Verification items for the finished model (mm, model axes). A direction names the side the tool comes from. Round coordinates to 2 decimals unless told otherwise and drop trailing zeros. Order: outer loops, then holes, each group sorted by start corner. A loop starts at its lowest first (then second) coordinate and runs counter-clockwise, first axis right, second up.
```python
from build123d import *

# Parameters (mm, degrees)
CROQUIS1_W              = 50
CROQUIS1_H              = 97
SALIENTE_EXTRUIR1_DEPTH = 5
CORTAR_EXTRUIR1_DEPTH   = 6
CROQUIS2_R              = 3.6
CROQUIS2_R_2            = 2.55
CORTAR_EXTRUIR2_DEPTH   = 6
CROQUIS4_R              = 6
CROQUIS4_R_2            = 5.05
CORTAR_EXTRUIR3_DEPTH   = 2
REDONDEO1_R             = 5
CROQUIS5_R              = 1.55
CROQUIS5_W              = 6
CROQUIS5_H              = 4.2
CORTAR_EXTRUIR4_DEPTH   = 6
CORTAR_EXTRUIR6_DEPTH   = 6
CROQUIS14_R             = 3
CORTAR_EXTRUIR9_DEPTH   = 2.5
CROQUIS18_R             = 10.5
CROQUIS18_R_2           = 1.525
CORTAR_EXTRUIR10_DEPTH  = 6


with BuildPart() as part:
    # Croquis1 → Saliente-Extruir1 (new body)
    with BuildSketch(Plane(origin=(0, 0, 0), x_dir=(1, 0, 0), z_dir=(0, 1, 0))):
        Rectangle(CROQUIS1_W, CROQUIS1_H)
    extrude(amount=SALIENTE_EXTRUIR1_DEPTH)

    # Croquis3 → Cortar-Extruir1 (cut, through all)
    with BuildSketch(Plane(origin=(0, 5, 0), x_dir=(1, 0, 0), z_dir=(0, 1, 0))):
        with BuildLine():
            Line((-14.1, -41.5), (-14.1, -48.5))
            Line((-14.1, -48.5), (-25, -48.5))
            Line((-25, -48.5), (-25, -28.05))
            ThreePointArc((-25, -28.05), (-17.369189497, -33.007651712), (-14.1, -41.5))
        make_face()
        with BuildLine():
            Line((25, -48.5), (14.1, -48.5))
            Line((14.1, -48.5), (14.1, -41.5))
            ThreePointArc((14.1, -41.5), (17.369189497, -33.007651712), (25, -28.05))
            Line((25, -28.05), (25, -48.5))
        make_face()
    extrude(amount=-CORTAR_EXTRUIR1_DEPTH, mode=Mode.SUBTRACT)

    # Croquis2 → Cortar-Extruir2 (cut, through all)
    with BuildSketch(Plane(origin=(0, 5, 0), x_dir=(1, 0, 0), z_dir=(0, 1, 0))):
        with Locations((-15, 32.45)):
            Circle(CROQUIS2_R)
        with Locations((15, 32.45)):
            Circle(CROQUIS2_R)
        with Locations((15, -19.45)):
            Circle(CROQUIS2_R_2)
        with Locations((-15, -19.45)):
            Circle(CROQUIS2_R_2)
    extrude(amount=-CORTAR_EXTRUIR2_DEPTH, mode=Mode.SUBTRACT)

    # Croquis4 → Cortar-Extruir3 (cut)
    with BuildSketch(Plane.XZ):
        with Locations((15, -32.45)):
            Circle(CROQUIS4_R)
        with Locations((-15, -32.45)):
            Circle(CROQUIS4_R)
        with Locations((-15, 19.45)):
            Circle(CROQUIS4_R_2)
        with Locations((15, 19.45)):
            Circle(CROQUIS4_R_2)
    extrude(amount=-CORTAR_EXTRUIR3_DEPTH, mode=Mode.SUBTRACT)

    # Redondeo1
    redondeo1_edges = [part.edges().sort_by_distance(p)[0] for p in [
        (-25, 2.5, 28.05),
        (25, 2.5, 28.05),
        (-25, 2.5, -48.5),
        (25, 2.5, -48.5),
    ]]
    fillet(redondeo1_edges, radius=REDONDEO1_R)

    # Croquis5 → Cortar-Extruir4 (cut, through all)
    with BuildSketch(Plane(origin=(0, 5, 0), x_dir=(1, 0, 0), z_dir=(0, 1, 0))):
        with Locations((0, 43.5)):
            Circle(CROQUIS5_R)
        with Locations((-11, 43.5)):
            Rectangle(CROQUIS5_W, CROQUIS5_H)
        with Locations((11, 43.5)):
            Rectangle(CROQUIS5_W, CROQUIS5_H)
    cortar_extruir4 = extrude(amount=-CORTAR_EXTRUIR4_DEPTH, mode=Mode.SUBTRACT)

    # Croquis8 → Cortar-Extruir6 (cut, through all)
    with BuildSketch(Plane(origin=(0, 5, 0), x_dir=(1, 0, 0), z_dir=(0, 1, 0))):
        with BuildLine():
            Line((-11.878679656, 45.6), (-10.121320344, 45.6))
            ThreePointArc((-10.121320344, 45.6), (-8.010608171, 45.610503119), (-7.979099854, 43.5))
            ThreePointArc((-7.979099854, 43.5), (-8.010608171, 41.389496881), (-10.121320344, 41.4))
            Line((-10.121320344, 41.4), (-11.878679656, 41.4))
            ThreePointArc((-11.878679656, 41.4), (-13.989391829, 41.389496881), (-14.020900146, 43.5))
            ThreePointArc((-14.020900146, 43.5), (-13.989391829, 45.610503119), (-11.878679656, 45.6))
        make_face()
        with BuildLine():
            Line((10.121320344, 41.4), (11.878679656, 41.4))
            ThreePointArc((11.878679656, 41.4), (13.989391829, 41.389496881), (14.020900146, 43.5))
            ThreePointArc((14.020900146, 43.5), (13.989391829, 45.610503119), (11.878679656, 45.6))
            Line((11.878679656, 45.6), (10.121320344, 45.6))
            ThreePointArc((10.121320344, 45.6), (8.010608171, 45.610503119), (7.979099854, 43.5))
            ThreePointArc((7.979099854, 43.5), (8.010608171, 41.389496881), (10.121320344, 41.4))
        make_face()
    cortar_extruir6 = extrude(amount=-CORTAR_EXTRUIR6_DEPTH, mode=Mode.SUBTRACT)

    # Simetría1: Cortar-Extruir4, Cortar-Extruir6 across plane
    add(cortar_extruir4.mirror(Plane.XY.offset(-26)), mode=Mode.SUBTRACT)
    add(cortar_extruir6.mirror(Plane.XY.offset(-26)), mode=Mode.SUBTRACT)

    # Croquis14 → Cortar-Extruir9 (cut)
    with BuildSketch(Plane(origin=(0, 5, 0), x_dir=(1, 0, 0), z_dir=(0, 1, 0))):
        with Locations((0, 8.5)):
            Circle(CROQUIS14_R)
    extrude(amount=-CORTAR_EXTRUIR9_DEPTH, mode=Mode.SUBTRACT)

    # Croquis18 → Cortar-Extruir10 (cut, through all)
    with BuildSketch(Plane(origin=(0, 5, 0), x_dir=(1, 0, 0), z_dir=(0, 1, 0))):
        with Locations((0, -35.5)):
            Circle(CROQUIS18_R)
        with Locations((9.75, -45.5)):
            Circle(CROQUIS18_R_2)
        with Locations((-9.75, -45.5)):
            Circle(CROQUIS18_R_2)
        with Locations((9.75, -25.5)):
            Circle(CROQUIS18_R_2)
        with Locations((-9.75, -25.5)):
            Circle(CROQUIS18_R_2)
    extrude(amount=-CORTAR_EXTRUIR10_DEPTH, mode=Mode.SUBTRACT)


solid = part.part
```
1) Go/stop test with flat-tipped pins: pin 1 Ø6 at (x, z) = (14, -35) entering from -Y; pin 2 Ø1.8 at (x, z) = (1, -8) entering from +Y. Record where each tip stops, or that it passes through.
2) Sectioned sample at B-B on x = 0. Record the cut outline in (y, z).
3) Scan lines: probe 1 along X at (y, z) = (3.6, 19.45); probe 2 along Z at (x, y) = (0, 1.75); probe 3 along Z at (x, y) = (0, 3.6). Record each from-to range of solid material in increasing order.
4) Tool access check on faces 1 (the flat face through (-11, 3, -45.6)), 2 (the flat face through (14, 2, 22)), 3 (the flat face through (1, 2.5, -7)), 4 (the flat face through (-14.1, 3, 45)). Record the directions out of +Z, -Z, +X, -X, +Y, -Y that give a thin tool (end or side, any length) a straight path to the whole face; none if there is none.
5) Sectioned sample at A-A on z = -32.45. Record the cut outline in (x, y).
6) Sectioned sample at C-C on x = -6. Record the cut outline in (y, z), then the cut area to 3 significant figures.
Returned:
1. pin 1: stops at y = 2
1. pin 2: stops at y = 2.5
2. outline: (0, -48.5) - (5, -48.5) - (5, -45.05) - (0, -45.05) - close; (0, -41.95) - (5, -41.95) - (5, -11.5) - (2.5, -11.5) - (2.5, -10.05) - (0, -10.05) - close; (0, -6.95) - (2.5, -6.95) - (2.5, -5.5) - (5, -5.5) - (5, 25) - (0, 25) - close; (0, 46) - (5, 46) - (5, 48.5) - (0, 48.5) - close
3. probe 1: x = -25 to -17.55, -12.45 to 12.45, 17.55 to 25
3. probe 2: z = -48.5 to -45.05, -41.95 to -10.05, -6.95 to 25, 46 to 48.5
3. probe 3: z = -48.5 to -45.05, -41.95 to -11.5, -5.5 to 25, 46 to 48.5
4. face 1: +Y, -Y
4. face 2: -Y
4. face 3: +Y
4. face 4: +Z, -X, +Y, -Y
5. outline: (-25, 0) - (-21, 0) - (-21, 2) - (-18.6, 2) - (-18.6, 5) - (-25, 5) - close; (-11.4, 2) - (-9, 2) - (-9, 0) - (9, 0) - (9, 2) - (11.4, 2) - (11.4, 5) - (-11.4, 5) - close; (18.6, 2) - (21, 2) - (21, 0) - (25, 0) - (25, 5) - (18.6, 5) - close
6. outline: (0, -48.5) - (5, -48.5) - (5, 26.88) - (0, 26.88) - close; (0, 44.12) - (5, 44.12) - (5, 48.5) - (0, 48.5) - close
6. area: 399 mm2
